Can you work these out from the model? Positions are in its coordinate system, mm. Coordinates: 2 decimals unless noted, no trailing zeros. Loops run counter-clockwise (first coordinate to the right, second up) from the corner with the lowest first, then second, coordinate; pieces in that order, holes last. Notation, with made-up numbers: (86.25, 80) -> (94.25, 80) arc R27 ccw to (94.25, 104) -> close; hole circle Ø11 at (29.5, 10.25). An arc over 180 degrees is marked (long way). Use one line per item in the form item = value. Start each with the question number.
(1) Imagine slicing it at B-B (z = 0). State how many separate pieces and enclosed holes the cut face has, plus the area to 3 significant figures.
(2) Imagine slicing it at A-A (x = -41). List the corners of the cut face in (y, z) for me.
(3) Thinking about a two-plate mould opening in Z: for faces 1 (the flat face through (-64.2, 30, -18)), 2 (the flat face through (-52, 30, -20)), 3 (the flat face through (-52, 30, 20)), 4 (the cylindrical face through (-44.2, 29.6, 0.3)), which applies, released by +Z, released by -Z, zero draft, split by the parting line, or undercut?
(4) Imagine slicing it at C-C (z = 16.5). List the corners of the cut face in (x, y) for me, plus the area to 3 significant figures.
(5) I need wall thicknesses on line 1 (Y direction, x = -51.75, z = 0); line 2 (Z direction, x = -46.25, y = 15); line 3 (Z direction, x = -40.75, y = 4.5). Which ranges of each line are inside material? Lowest first, please. Write a range as [from, to].
(6) I'm going to push flat-ended pins straight in: pin 1 (7 mm diameter, centred on y = 15, z = 0, fed in from +X); pin 2 (5 mm diameter, centred on y = 45, z = 0, fed in from -X); pin 3 (8 mm diameter, centred on x = -55.5, z = 5.5, fed in from -Y); pin 4 (2 mm diameter, centred on y = 23.5, z = 0.5, fed in from +X). Where does each tip first touch, or does it pass through?
```python
from build123d import *

# Parameters (mm, degrees)
BOSS_EXTRUDE1_DEPTH      = 60
M4_CLEARANCE_HOLE1_D     = 4.5
M4_CLEARANCE_HOLE1_DEPTH = 70
M4_CLEARANCE_HOLE1_TIP   = 1.351936393


with BuildPart() as part:
    # Sketch1 → Boss-Extrude1 (new body)
    with BuildSketch(Plane(origin=(0, 0, 0), x_dir=(1, 0, 0), z_dir=(0, 1, 0))):
        with BuildLine():
            Line((-64.199832154, 20), (-64.199832154, 15))
            add(Edge.make_bspline(
                [(-64.199832154, -15), (-54.199832154, -15), (-54.199832154, 0), (-54.199832154, 15), (-64.199832154, 15)],
                knots=[3.141592654, 3.141592654, 3.141592654, 4.71238898, 4.71238898, 6.283185307, 6.283185307, 6.283185307], degree=2, weights=[1, 0.707106781, 1, 0.707106781, 1]))
            Line((-64.199832154, -15), (-64.199832154, -20))
            Line((-64.199832154, -20), (-39.416052091, -20))
            ThreePointArc((-39.416052091, -20), (-44.199832154, 0), (-39.416052091, 20))
            Line((-39.416052091, 20), (-64.199832154, 20))
        make_face()
    extrude(amount=BOSS_EXTRUDE1_DEPTH)

    # M4 Clearance Hole1
    with Locations(Plane(origin=(0, 0, 0), x_dir=(0, 0, -1), z_dir=(1, 0, 0))):
        with Locations((0, 45), (0, 15)):
            Hole(M4_CLEARANCE_HOLE1_D / 2, depth=M4_CLEARANCE_HOLE1_DEPTH)
            with Locations((0, 0, -(M4_CLEARANCE_HOLE1_DEPTH + M4_CLEARANCE_HOLE1_TIP / 2))):  # 118° drill point
                Cone(0, M4_CLEARANCE_HOLE1_D / 2, M4_CLEARANCE_HOLE1_TIP, mode=Mode.SUBTRACT)


solid = part.part
```
Worked out:
q1.separate_pieces = 3
q1.enclosed_holes = 0
q1.area = 510 mm2
q2.outline = (0, -20) -> (60, -20) -> (60, -16.51) -> (0, -16.51) -> close; (0, 16.51) -> (60, 16.51) -> (60, 20) -> (0, 20) -> close
q3.face_1 = zero draft
q3.face_2 = released by -Z
q3.face_3 = released by +Z
q3.face_4 = undercut
q4.outline = (-64.2, 0) -> (-41, 0) -> (-41, 60) -> (-64.2, 60) -> close
q4.area = 1,390 mm2
q5.line_1 = [0, 12.75], [17.25, 42.75], [47.25, 60]
q5.line_2 = [-20, -2.25], [2.25, 20]
q5.line_3 = [-20, -17.12], [17.12, 20]
q6.pin_1 = -44.06
q6.pin_2 = -54.34
q6.pin_3 = 0
q6.pin_4 = -44.17
